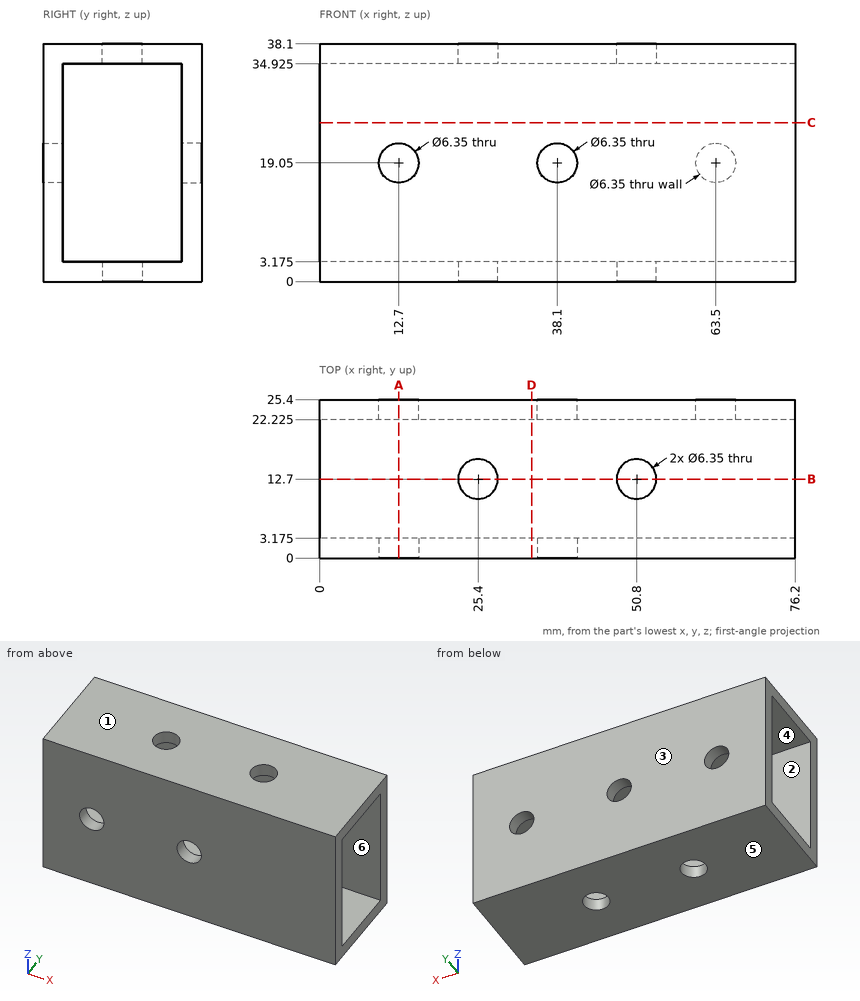
Job drawing, mm, ordinate dimensions from the low corner. One solid piece. A direction names the side the tool comes from. Coordinates: 2 decimals unless noted, no trailing zeros. Order: outer loops, then holes, each group sorted by start corner. A loop starts at its lowest first (then second) coordinate and runs counter-clockwise, first axis right, second up. Notation, with made-up numbers: M 25.5,-11 L 81.5,-11 A30 cw 81.5,26 Z; hole C 49,42.25 d8. An arc over 180 degrees is marked long. One line per question, with ' | ' between items.
Q1. Drill centre lines: line 1 (X direction, y = 24.3, z = 19.05) (3 decimals); line 2 (Z direction, x = 46, y = 12.5) (3 decimals); line 3 (Y direction, x = 51.5, z = 25.5) (3 decimals). Where is each one in solid material? Low to high.
A:
line 1: x = 0 to 9.525, 15.875 to 34.925, 41.275 to 60.325, 66.675 to 76.2 | line 2: z = 0 to 3.175, 34.925 to 38.1 | line 3: y = 0 to 3.175, 22.225 to 25.4
Q2. Slice it at A-A (x = 12.7). Give the cut face in (y, z) (3 decimals), and give its area (3 significant figures).
A:
outline: M 0,0 L 25.4,0 L 25.4,15.875 L 22.225,15.875 L 22.225,3.175 L 3.175,3.175 L 3.175,15.875 L 0,15.875 Z; M 0,22.225 L 3.175,22.225 L 3.175,34.925 L 22.225,34.925 L 22.225,22.225 L 25.4,22.225 L 25.4,38.1 L 0,38.1 Z | area: 323 mm^2
Q3. Two-plate mould, pull along Z, no slides. Class the marked faces 3, 4, 5 and 6: +Z half, -Z half, draft (parallel to the pull), parting line (faces both ways), or undercut.
A:
face 3: draft | face 4: undercut | face 5: -Z half | face 6: undercut
Q4. Slice it at D-D (x = 34). Give the cut face in (y, z) (3 decimals), and give its area (3 significant figures).
A:
outline: M 0,0 L 25.4,0 L 25.4,38.1 L 0,38.1 Z; hole M 3.175,3.175 L 22.225,3.175 L 22.225,34.925 L 3.175,34.925 Z | area: 363 mm^2
Q5. Slice it at B-B (y = 12.7). Give the cut face in (x, z) (3 decimals), and give its area (3 significant figures).
A:
outline: M 0,0 L 22.225,0 L 22.225,3.175 L 0,3.175 Z; M 0,34.925 L 22.225,34.925 L 22.225,38.1 L 0,38.1 Z; M 28.575,0 L 47.625,0 L 47.625,3.175 L 28.575,3.175 Z; M 28.575,34.925 L 47.625,34.925 L 47.625,38.1 L 28.575,38.1 Z; M 53.975,0 L 76.2,0 L 76.2,3.175 L 53.975,3.175 Z; M 53.975,34.925 L 76.2,34.925 L 76.2,38.1 L 53.975,38.1 Z | area: 403 mm^2
Q6. Slice it at C-C (z = 25.5). Give the cut face in (x, y) (3 decimals).
A:
outline: M 0,0 L 76.2,0 L 76.2,3.175 L 0,3.175 Z; M 0,22.225 L 76.2,22.225 L 76.2,25.4 L 0,25.4 Z
Q7. 3-axis set-ups, long thin cutter, end or side, ignore diameter. For the marked faces 1 and 2: which of +Z, -Z, +X, -X, +Y, -Y reach the whole face in a straight line?
A:
face 1: +Z, +X, -X, +Y, -Y | face 2: +X, -X
